Verification items for this drawing (mm, ordinates from the low corner). Coordinates: 2 decimals unless noted, no trailing zeros. Write each loop counter-clockwise with the first axis right and the second up, starting at its lowest first coordinate (ties: lowest second). Pieces come first, ordered by that corner, then holes. Notation, with made-up numbers: (88, -1.5) -> (106, -1.5) arc R30 cw to (106, 32.5) -> close; hole circle Ø9 at (-9.5, -1.75). An arc over 180 degrees is marked (long way). Put each result on its own line as item: value. Start each with the question number.
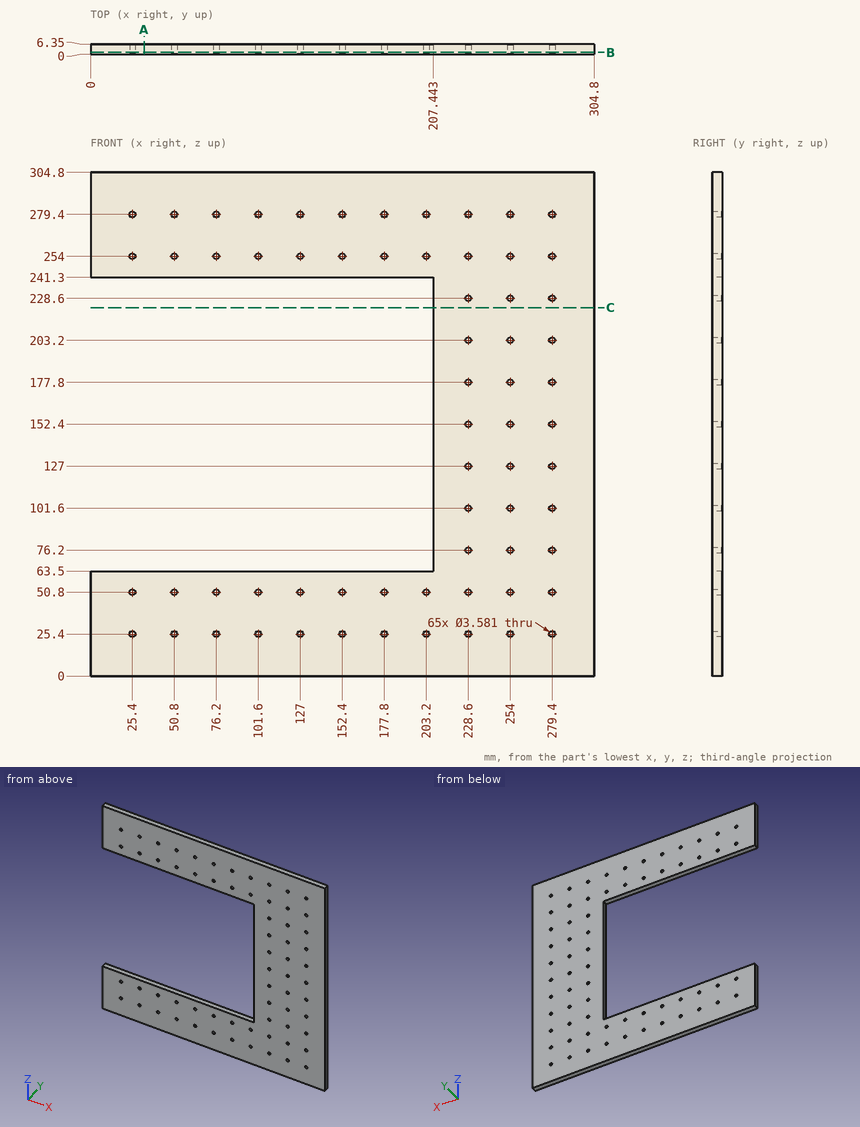
Item 1: Go/stop test with a flat-tipped pin: P1, Ø3, axis at x = 76.2, z = 254, coming from the -Y side. Record where the tip stops, or that it passes through.
Item 2: Section check A-A, the plane x = 32.5. Enter the section's corners in (y, z).
Item 3: Section check C-C, the plane z = 223. Enter the section's corners in (x, y), and give its area (3 significant figures).
Item 4: Section check B-B, the plane y = 1.25. Give the number of separate pieces and of enclosed holes in the cut face, and give its area (3 significant figures).
Item 5: Scan lines: line 1 along Z through (x, y) = (177.8, 4.25); line 2 along Z through (x, y) = (167, 3.5); line 3 along X through (y, z) = (1.5, 228.6). Record each from-to range of solid material in increasing order. Write a range as [from, to].
From the geometry:
1. P1: through
2. outline: (0, 0) -> (6.35, 0) -> (6.35, 63.5) -> (0, 63.5) -> close; (0, 241.3) -> (6.35, 241.3) -> (6.35, 304.8) -> (0, 304.8) -> close
3. outline: (207.44, 0) -> (304.8, 0) -> (304.8, 6.35) -> (207.44, 6.35) -> close
3. area: 618 mm²
4. separate pieces: 1
4. enclosed holes: 65
4. area: 55,400 mm²
5. line 1: [0, 23.61], [27.19, 49.01], [52.59, 63.5], [241.3, 252.21], [255.79, 277.61], [281.19, 304.8]
5. line 2: [0, 63.5], [241.3, 304.8]
5. line 3: [207.44, 226.81], [230.39, 252.21], [255.79, 277.61], [281.19, 304.8]
